from build123d import *

# Parameters (mm, degrees)
SKETCH2_R           = 51
BOSS_EXTRUDE1_DEPTH = 102
SKETCH3_R           = 75
BOSS_EXTRUDE2_DEPTH = 102
BOSS_EXTRUDE3_DEPTH = 102
BOSS_EXTRUDE7_START = 100
SKETCH17_R          = 38
BOSS_EXTRUDE7_DEPTH = 75


with BuildPart() as part:
    # Sketch2 → Boss-Extrude1 (new body)
    with BuildSketch(Plane.XY.offset(355)):
        with BuildLine():
            Line((-285, 765), (0, 765))
            Line((0, 765), (0, 0))
            Line((0, 0), (-595, 0))
            ThreePointArc((-595, 0), (-687.466864274, 55.251844141), (-682.620113823, 162.859447402))
            Line((-682.620113823, 162.859447402), (-285, 765))
        make_face()
        with Locations((-595, 105)):
            Circle(SKETCH2_R, mode=Mode.SUBTRACT)
    boss_extrude1 = extrude(amount=BOSS_EXTRUDE1_DEPTH)

    # Sketch3 → Boss-Extrude2 (add)
    with BuildSketch(Plane(origin=(0, 765, 0), x_dir=(1, 0, 0), z_dir=(0, 1, 0))):
        with BuildLine():
            Line((0, -457), (-285, -457))
            Line((-285, -457), (-285, 253))
            Line((-285, 253), (0, 253))
            Line((0, 253), (322.019203343, 78.15740693))
            ThreePointArc((322.019203343, 78.15740693), (429.201471167, -102), (322.019203343, -282.15740693))
            Line((322.019203343, -282.15740693), (0, -457))
        make_face()
        with Locations((224.201471167, -102)):
            Circle(SKETCH3_R, mode=Mode.SUBTRACT)
    extrude(amount=-BOSS_EXTRUDE2_DEPTH)

    # Mirror2: Boss-Extrude1 across plane
    add(boss_extrude1.mirror(Plane.XY.offset(102)))

    # Sketch9 → Boss-Extrude3 (add)
    with BuildSketch(Plane.XZ):
        with BuildLine():
            Line((0, -151), (0, -253))
            Line((0, -253), (322.019203343, -78.15740693))
            ThreePointArc((322.019203343, -78.15740693), (429.201471167, 102), (322.019203343, 282.15740693))
            Line((322.019203343, 282.15740693), (0, 457))
            Line((0, 457), (0, 355))
            Line((0, 355), (-285, 355))
            Line((-285, 355), (-285, -151))
            Line((-285, -151), (0, -151))
        make_face()
    extrude(amount=-BOSS_EXTRUDE3_DEPTH)

    # Sketch17 → Boss-Extrude7 (add)
    with BuildSketch(Plane.XY.offset(102).offset(BOSS_EXTRUDE7_START)):
        with BuildLine():
            Line((-234.97331208, 765), (0, 765))
            Line((0, 765), (-220.558080551, 1027.850884872))
            ThreePointArc((-220.558080551, 1027.850884872), (-347.352965303, 1038.943999881), (-358.446080312, 912.149115128))
            Line((-358.446080312, 912.149115128), (-234.97331208, 765))
        make_face()
        with Locations((-289.502080431, 970)):
            Circle(SKETCH17_R, mode=Mode.SUBTRACT)
    boss_extrude7 = extrude(amount=BOSS_EXTRUDE7_DEPTH)

    # Mirror5: Boss-Extrude7 across plane
    add(boss_extrude7.mirror(Plane.XY.offset(102)))


solid = part.part
Can you work these out from the model? Positions are in its coordinate system, mm. A direction names the side the tool comes from. Give positions to 0.01 mm unless a question says otherwise; leave off trailing zeros. Loops run counter-clockwise (first coordinate to the right, second up) from the corner with the lowest first, then second, coordinate; pieces in that order, holes last. Notation, with made-up numbers: (66.25, 29) - (78.25, 29) arc R20 ccw to (78.25, 66) - close; hole circle Ø3 at (53, 36.25). An arc over 180 degrees is marked (long way). One line per item, written item: value.
(1) I need wall thicknesses on line 1 along Y through (x, z) = (325, 6); line 2 along Z through (x, y) = (-5, 540.5); line 3 along X through (y, z) = (534, -184.5). Which ranges of each line are inside material? Lowest first, please.
Verdict:
line 1: 0 to 102, 663 to 765
line 2: -253 to -151, 355 to 457
line 3: -437.54 to 0
(2) On a 3-axis mill with a long thin cutter (end or side, diameter ignored), from which of +Z, -Z, +X, -X, +Y, -Y can I reach the whole of each face in a straight line? I mean faces 5 (the face through (-285, 715, 106)), 6 (the face through (0, 386, 405)), 7 (the face through (429.18, 50.29, 98.92)), 8 (the face through (164.684, 714.714, 147.636)), 9 (the face through (-235, 882, -73)). Say none if no direction works.
Verdict:
face 5: -X, -Y
face 6: +Z, -Z, +X
face 7: +X, +Y, -Y
face 8: +Y
face 9: -Z, +X, -X, +Y
(3) If we section it at D-D, the plane x = 112: List the corners of the cut face in (y, z) for me.
Verdict:
outline: (0, -192.19) - (102, -192.19) - (102, 396.19) - (0, 396.19) - close; (663, -192.19) - (765, -192.19) - (765, 396.19) - (663, 396.19) - close
(4) If we section it at C-C, the plane z = -100.5: List the corners of the cut face in (x, y) for me, plus the area to 3 significant figures.
Verdict:
outline: (-285, 0) - (280.87, 0) - (280.87, 102) - (-285, 102) - close; (-285, 663) - (280.87, 663) - (280.87, 765) - (-285, 765) - close
area: 115,000 mm^2
(5) If we section it at A-A, the plane z = 102: List the corners of the cut face in (x, y) for me, plus the area to 3 significant figures.
Verdict:
outline: (-285, 0) - (429.2, 0) - (429.2, 102) - (-285, 102) - close; (-285, 663) - (149.2, 663) - (149.2, 765) - (-285, 765) - close; (299.2, 663) - (429.2, 663) - (429.2, 765) - (299.2, 765) - close
area: 130,000 mm^2
(6) If we mould it in two halves opening along Z, with no side actions, what happens to faces 1 (the face through (-267, 303, 457)), 2 (the face through (-235, 882, 2)), 3 (the face through (158.76, 714.71, -166.8)), 4 (the face through (-108.74, 894.59, 238.98))? For each: released by +Z, released by -Z, zero draft, split by the parting line, or undercut.
Verdict:
face 1: released by +Z
face 2: undercut
face 3: released by -Z
face 4: zero draft
(7) If we section it at B-B, the plane y = 970: List the corners of the cut face in (x, z) for me, plus the area to 3 significant figures.
Verdict:
outline: (-379.5, -73) - (-327.5, -73) - (-327.5, 2) - (-379.5, 2) - close; (-379.5, 202) - (-327.5, 202) - (-327.5, 277) - (-379.5, 277) - close; (-251.5, -73) - (-172.02, -73) - (-172.02, 2) - (-251.5, 2) - close; (-251.5, 202) - (-172.02, 202) - (-172.02, 277) - (-251.5, 277) - close
area: 19,700 mm^2
